```python
from build123d import *

# Parameters (mm, degrees)
F0_W          = 100
F0_H          = 100
F1_DEPTH      = 50
F3_DEPTH      = 100
F5_DEPTH      = 100
F5_DEPTH_BACK = 100


with BuildPart() as f1:
    # F0 (on Top) → F1 (new body, symmetric)
    with BuildSketch(Plane.XY):
        Rectangle(F0_W, F0_H)
    extrude(amount=F1_DEPTH, both=True)

    # F2 (on face) → F3 (cut, through all)
    with BuildSketch(Plane.YZ.offset(50)):
        Polygon((-50, -50), (0, -50), (-50, 50), align=None)
        Polygon((50, -50), (50, 50), (0, -50), align=None)
    extrude(amount=-F3_DEPTH, mode=Mode.SUBTRACT)

    # F4 (on Front) → F5 (cut, two sides)
    with BuildSketch(Plane.XZ) as f5_sk:
        Polygon((50, 50), (0, -50), (50, -50), align=None)
        Polygon((0, -50), (-50, 50), (-50, -50), align=None)
    extrude(amount=-F5_DEPTH, mode=Mode.SUBTRACT)
    extrude(f5_sk.sketch, amount=F5_DEPTH_BACK, mode=Mode.SUBTRACT)


solid = f1.part
```
Can you work these out from the model? Positions are in its coordinate system, mm. Give positions to 0.01 mm unless a question says otherwise; leave off trailing zeros. Loops run counter-clockwise (first coordinate to the right, second up) from the corner with the lowest first, then second, coordinate; pieces in that order, holes last. Notation, with made-up numbers: M -36.5,20 L -22.5,20 A22 cw -22.5,27 Z; hole C 11,7.5 d3. An arc over 180 degrees is marked long. Use CSV: the item, a comma, the result in double quotes. Start each with the question number.
1. For P1, Ø8, axis at x = 4.5, z = 22.5, coming from the +Y side; P2, Ø12, axis at x = 13.5, z = 19, coming from the -Y side; P3, Ø6, axis at x = -26, y = 19.5, coming from the -Z side, each with a flat end and sliding along its axis, tell me the tip position at first contact or that it passes through.
2. If I drill on L1, parallel to Z at x = 6, y = -26.5; L2, parallel to X at y = -23.5, z = 43; L3, parallel to Y at x = -22, z = 3, over which ranges is the centre line in solid material (lowest first)?
3. If we mould it in two halves opening along X, with no side actions, what happens to faces 1 (the face through (-30, 1, 10)), 2 (the face through (31, 1, 12)), 3 (the face through (1, -30, 10))? For each: released by +X, released by -X, zero draft, split by the parting line, or undercut.
4. Imagine slicing it at A-A, the plane z = -1.5. Write out the boundary of the cut face in (x, y), plus the area to 3 significant figures.
5. Imagine slicing it at B-B, the plane x = 3. Write out the boundary of the cut face in (y, z), plus the area to 3 significant figures.
Response values:
1,P1,"y = 38.25"
1,P2,"y = -37.5"
1,P3,"z = -4"
2,L1,"3 to 50"
2,L2,"-46.5 to 46.5"
2,L3,"-26.5 to 26.5"
3,face 1,"released by -X"
3,face 2,"released by +X"
3,face 3,"zero draft"
4,outline,"M -24.25,-24.25 L 24.25,-24.25 L 24.25,24.25 L -24.25,24.25 Z"
4,area,"2,350 mm^2"
5,outline,"M -50,50 L -3,-44 L 3,-44 L 50,50 Z"
5,area,"4,980 mm^2"
